Source: CAD feature listing. Evaluate the final solid. Frame: model axes, mm. A direction names the side the tool comes from. Round coordinates to 2 decimals unless told otherwise and drop trailing zeros. Order: outer loops, then holes, each group sorted by start corner. A loop starts at its lowest first (then second) coordinate and runs counter-clockwise, first axis right, second up. Notation, with made-up numbers: (-15, 19) - (3, 19) arc R13 cw to (3, 32) - close; hole circle Ø5 at (8.5, -24.5). An arc over 180 degrees is marked (long way). Put each result on its own line as item: value. Start each with the question number.
1) Section A-A on y = -20.25. Output: boundary loops of the cut face in (x, z).
2) Section C-C on z = -5.25. Output: boundary loops of the cut face in (x, y).
3) Contact query for flat-ended pins moving along their axis: P1, Ø2, axis at x = -5, z = 1.5, coming from the -Y side; P2, Ø0.5, axis at x = -2.5, y = -20.5, coming from the -Z side; P3, Ø0.6, axis at y = -21.5, z = -0.5, coming from the +X side; P4, Ø5, axis at y = -21, z = 7, coming from the +X side. Output: stop coordinate, or through.
4) Section B-B on x = 0. Output: boundary loops of the cut face in (y, z), then the cut area to 3 significant figures.
5) Line query: probe 1 along Z at (x, y) = (2.75, -19.25); probe 2 along X at (y, z) = (-19.5, -1); probe 3 along X at (y, z) = (-20.75, -6). Output: solid intervals per line, ascending. Write a range as [from, to].
6) Section D-D on y = -4.5. Output: boundary loops of the cut face in (x, z), then the cut area to 3 significant figures.
7) Access query for faces 4 (the face through (2.222, -21, -1)), 5 (the face through (6.323, 3.538, 1.404)), 6 (the face through (2.858, -21, -1)), 7 (the face through (3.302, -21, -5)), 8 (the face through (-8, 0, 0)). Directions: +Z, -Z, +X, -X, +Y, -Y. A direction counts if a zero-diameter tool reaches every point of the face in a straight line with its end or side. Return the directions, or none.
8) Mould query, pull axis X, two halves, no side actions, for faces 1 (the face through (8.954, 1, 0)), 2 (the face through (0, 1, 8.954)), 3 (the face through (-2.667, -21, -5)). Classes: +X half, -X half, draft (parallel to the pull), parting line (faces both ways), or undercut.
```python
from build123d import *

# Parameters (mm, degrees)
SKETCH1_W           = 17.907
SKETCH1_H           = 17.907
BOSS_EXTRUDE1_DEPTH = 2.286
SKETCH2_R           = 6.477
BOSS_EXTRUDE2_DEPTH = 2.54
SKETCH3_R           = 7.8232
BOSS_EXTRUDE3_DEPTH = 18.288
SKETCH4_W           = 0.635
SKETCH4_H           = 2.0574
BOSS_EXTRUDE4_DEPTH = 6.096


with BuildPart() as part:
    # Sketch1 → Boss-Extrude1 (new body)
    with BuildSketch(Plane(origin=(0, 0, 0), x_dir=(1, 0, 0), z_dir=(0, 1, 0))):
        Rectangle(SKETCH1_W, SKETCH1_H)
    extrude(amount=BOSS_EXTRUDE1_DEPTH)

    # Sketch2 → Boss-Extrude2 (add)
    with BuildSketch(Plane(origin=(0, 2.286, 0), x_dir=(1, 0, 0), z_dir=(0, 1, 0))):
        with Locations(Location((0, 0, 0), (0, 0, 90))):  # turned: the seam where the file's is
            Circle(SKETCH2_R)
    extrude(amount=BOSS_EXTRUDE2_DEPTH)

    # Sketch3 → Boss-Extrude3 (add)
    with BuildSketch(Plane.XZ):
        with Locations(Location((0, 0, 0), (0, 0, 270))):  # turned: the seam where the file's is
            Circle(SKETCH3_R)
    extrude(amount=BOSS_EXTRUDE3_DEPTH)

    # Sketch4 → Boss-Extrude4 (add)
    with BuildSketch(Plane.XZ.offset(18.288)):
        with Locations((-2.54, -1.0287)):
            Rectangle(SKETCH4_W, SKETCH4_H)
        with Locations((2.54, -1.0287)):
            Rectangle(SKETCH4_W, SKETCH4_H)
        with Locations((-2.9845, -5.3213)):
            Rectangle(SKETCH4_W, SKETCH4_H)
        with Locations((2.9845, -5.3213)):
            Rectangle(SKETCH4_W, SKETCH4_H)
    extrude(amount=BOSS_EXTRUDE4_DEPTH)


solid = part.part
```
Answer sheet:
1. outline: (-3.3, -6.35) - (-2.67, -6.35) - (-2.67, -4.29) - (-3.3, -4.29) - close; (-2.86, -2.06) - (-2.22, -2.06) - (-2.22, 0) - (-2.86, 0) - close; (2.22, -2.06) - (2.86, -2.06) - (2.86, 0) - (2.22, 0) - close; (2.67, -6.35) - (3.3, -6.35) - (3.3, -4.29) - (2.67, -4.29) - close
2. outline: (-8.95, 0) - (-5.8, 0) - (-5.8, -18.29) - (-3.3, -18.29) - (-3.3, -24.38) - (-2.67, -24.38) - (-2.67, -18.29) - (2.67, -18.29) - (2.67, -24.38) - (3.3, -24.38) - (3.3, -18.29) - (5.8, -18.29) - (5.8, 0) - (8.95, 0) - (8.95, 2.29) - (3.79, 2.29) - (3.79, 4.83) - (-3.79, 4.83) - (-3.79, 2.29) - (-8.95, 2.29) - close
3. P1: y = -18.29
3. P2: z = -6.35
3. P3: x = 2.86
3. P4: through
4. outline: (-18.29, -7.82) - (0, -7.82) - (0, -8.95) - (2.29, -8.95) - (2.29, -6.48) - (4.83, -6.48) - (4.83, 6.48) - (2.29, 6.48) - (2.29, 8.95) - (0, 8.95) - (0, 7.82) - (-18.29, 7.82) - close
4. area: 360 mm^2
5. probe 1: [-6.35, -4.29], [-2.06, 0]
5. probe 2: [-2.86, -2.22], [2.22, 2.86]
5. probe 3: [-3.3, -2.67], [2.67, 3.3]
6. outline: circle Ø15.65 at (0, 0)
6. area: 192 mm^2
7. face 4: +Z, -Z, -Y
7. face 5: +Y
7. face 6: +Z, +X, -Y
7. face 7: +Z, -Z, +X, -Y
7. face 8: -Y
8. face 1: +X half
8. face 2: draft
8. face 3: undercut
